Geometry check sheet. Reference: the model listing, model coordinates, mm. A direction names the side the tool comes from. Coordinates: 2 decimals unless noted, no trailing zeros. Order: outer loops, then holes, each group sorted by start corner. A loop starts at its lowest first (then second) coordinate and runs counter-clockwise, first axis right, second up. Notation, with made-up numbers: (64.25, 56.25) - (94.25, 56.25) arc R25 cw to (94.25, 91.25) - close; hole circle Ø11 at (12, 77). An arc over 180 degrees is marked (long way). One line per item, written item: value. Start each with the question number.
```python
from build123d import *

# Parameters (mm, degrees)
MODEL_R             = 3.5
EXTRUDE_1_DEPTH     = 40
SKETCH_3_W          = 37
SKETCH_3_H          = 37
CUT_EXTRUDE_1_DEPTH = 40
SKETCH_4_R          = 1.5
CUT_EXTRUDE_2_DEPTH = 40
CUT_EXTRUDE1_REACH  = 42
SKETCH2_R           = 1.5


with BuildPart() as part:
    # Model → 凸台-拉伸1 (new body)
    with BuildSketch(Plane.XY):
        with BuildLine():
            Line((2619.766714505, 1592.826425633), (2619.766714505, 1609.326425633))
            Line((2619.766714505, 1609.326425633), (2592.766714505, 1609.326425633))
            Line((2592.766714505, 1609.326425633), (2592.766714505, 1592.826425633))
            ThreePointArc((2592.766714505, 1592.826425633), (2606.266714505, 1579.326425633), (2619.766714505, 1592.826425633))
        make_face()
        with Locations((2606.266714505, 1592.826425633)):
            Circle(MODEL_R, mode=Mode.SUBTRACT)
    extrude(amount=EXTRUDE_1_DEPTH)

    # 草图3 → 切除-拉伸1 (cut)
    with BuildSketch(Plane(origin=(2619.766714505, 0, 0), x_dir=(0, 0, -1), z_dir=(1, 0, 0))):
        with Locations((-21.5, 1587.826425633)):
            Rectangle(SKETCH_3_W, SKETCH_3_H)
    extrude(amount=-CUT_EXTRUDE_1_DEPTH, mode=Mode.SUBTRACT)

    # 草图4 → 切除-拉伸2 (cut)
    with BuildSketch(Plane(origin=(0, 1609.326425633, 0), x_dir=(1, 0, 0), z_dir=(0, 1, 0))):
        with Locations((2600.766714505, -32)):
            Circle(SKETCH_4_R)
        with Locations((2611.766714505, -32)):
            Circle(SKETCH_4_R)
        with Locations((2600.766714505, -12)):
            Circle(SKETCH_4_R)
        with Locations((2611.766714505, -12)):
            Circle(SKETCH_4_R)
    extrude(amount=-CUT_EXTRUDE_2_DEPTH, mode=Mode.SUBTRACT)

    # Sketch2 → Cut-Extrude1 (cut, up to next)
    with BuildSketch(Plane(origin=(0, 0, 0), x_dir=(-1, 0, 0), z_dir=(0, 0, -1)), mode=Mode.PRIVATE) as cut_extrude1_sk1:
        with Locations((-2597.766714505, 1592.826425633)):
            Circle(SKETCH2_R)
    cut_extrude1_tool1 = extrude(cut_extrude1_sk1.sketch, amount=-CUT_EXTRUDE1_REACH, mode=Mode.PRIVATE) & part.part
    add(cut_extrude1_tool1.solids().sort_by_distance((2597.766715, 1592.826426, 0))[0], mode=Mode.SUBTRACT)
    # Sketch2 → Cut-Extrude1 (cut, up to next)
    with BuildSketch(Plane(origin=(0, 0, 0), x_dir=(-1, 0, 0), z_dir=(0, 0, -1)), mode=Mode.PRIVATE) as cut_extrude1_sk2:
        with Locations((-2614.766714505, 1592.826425633)):
            Circle(SKETCH2_R)
    cut_extrude1_tool2 = extrude(cut_extrude1_sk2.sketch, amount=-CUT_EXTRUDE1_REACH, mode=Mode.PRIVATE) & part.part
    add(cut_extrude1_tool2.solids().sort_by_distance((2614.766715, 1592.826426, 0))[0], mode=Mode.SUBTRACT)


solid = part.part
```
Q1. Cross-section at B-B, the plane x = 2607.25. Enter the section's corners in (y, z), and give its area (3 significant figures).
Q2. Material ranges on probe 1 along X at (y, z) = (1607.1, 12); probe 2 along Z at (x, y) = (2611, 1592); probe 3 along Y at (x, z) = (2609, 16), recorded low to high.
Q3. Cross-section at A-A, the plane z = 32. Enter the section's corners in (x, y), and give its area (3 significant figures).
Q4. Cross-section at C-C, the plane y = 1595.5. Enter the section's corners in (x, z).
Q5. Set-up check for faces 4 (the cylindrical face through (2614.07, 1591.5, 1.48)), 5 (the flat face through (2603, 1596, 3)): record each of +Z, -Z, +X, -X, +Y, -Y from which the full face is reachable in a straight line by a thin tool's end or side.
Q6. Release check for a two-part mould opening along Y. For faces 1 (the cylindrical face through (2605.97, 1579.33, 1.48)), 2 (the flat face through (2592.767, 1607, 15)), 3 (the cylindrical face through (2602.77, 1592.98, 1.48)) record: released by +Y, released by -Y, zero draft, split by the parting line, or undercut.
Q7. Gauge pin test, flat ends, axial feed: P1, Ø2.5, axis at x = 2597.77, y = 1592.83, coming from the +Z side; P2, Ø1.5, axis at x = 2609.5, y = 1586.5, coming from the +Z side; P3, Ø2, axis at x = 2614.5, z = 15.5, coming from the -Y side. Record the tip position at first contact, or that the pin passes through.
Q8. Cross-section at D-D, the plane x = 2611. Enter the section's corners in (y, z).
Check result:
1. outline: (1579.36, 0) - (1589.47, 0) - (1589.47, 3) - (1579.36, 3) - close; (1596.19, 0) - (1609.33, 0) - (1609.33, 40) - (1606.33, 40) - (1606.33, 3) - (1596.19, 3) - close
1. area: 181 mm2
2. probe 1: x = 2592.77 to 2599.27, 2602.27 to 2610.27, 2613.27 to 2619.77
2. probe 2: z = 0 to 3
2. probe 3: y = 1606.33 to 1609.33
3. outline: (2592.77, 1606.33) - (2599.27, 1606.33) - (2599.27, 1609.33) - (2592.77, 1609.33) - close; (2602.27, 1606.33) - (2610.27, 1606.33) - (2610.27, 1609.33) - (2602.27, 1609.33) - close; (2613.27, 1606.33) - (2619.77, 1606.33) - (2619.77, 1609.33) - (2613.27, 1609.33) - close
3. area: 63.0 mm2
4. outline: (2592.77, 0) - (2604.01, 0) - (2604.01, 3) - (2592.77, 3) - close; (2608.53, 0) - (2619.77, 0) - (2619.77, 3) - (2608.53, 3) - close
5. face 4: +Z, -Z
5. face 5: +Z, +X, -X, -Y
6. face 1: released by -Y
6. face 2: zero draft
6. face 3: undercut
7. P1: passes through
7. P2: stops at z = 3
7. P3: stops at y = 1606.33
8. outline: (1580.18, 0) - (1609.33, 0) - (1609.33, 10.71) - (1606.33, 10.71) - (1606.33, 3) - (1580.18, 3) - close; (1606.33, 13.29) - (1609.33, 13.29) - (1609.33, 30.71) - (1606.33, 30.71) - close; (1606.33, 33.29) - (1609.33, 33.29) - (1609.33, 40) - (1606.33, 40) - close
